from build123d import *

# Parameters (mm, degrees)
F0_W     = 12
F0_H     = 12
F1_DEPTH = 75
F2_R     = 3.6
F3_DEPTH = 80
F4_R     = 0.6


with BuildPart() as f1:
    # F0 (on Top) → F1 (new body)
    with BuildSketch(Plane.XY):
        Rectangle(F0_W, F0_H)
    extrude(amount=F1_DEPTH)

    # F2 (on face) → F3 (cut)
    with BuildSketch(Plane.XY.offset(75)):
        Circle(F2_R)
    extrude(amount=-F3_DEPTH, mode=Mode.SUBTRACT)

    # F4
    f4_edges = [f1.edges().sort_by_distance(p)[0] for p in [
        (-6, -6, 37.5),
        (6, -6, 37.5),
        (0, -6, 0),
        (0, -6, 75),
        (6, 6, 37.5),
        (6, 0, 0),
        (6, 0, 75),
        (-6, 6, 37.5),
        (0, 6, 0),
        (0, 6, 75),
        (-6, 0, 0),
        (-6, 0, 75),
    ]]
    fillet(f4_edges, radius=F4_R)


solid = f1.part
Read the model definition and answer for the solid it produces. Units are mm, in the model's axes. Coordinates: 2 decimals unless noted, no trailing zeros. Order: outer loops, then holes, each group sorted by start corner. A loop starts at its lowest first (then second) coordinate and runs counter-clockwise, first axis right, second up. Notation, with made-up numbers: (75.25, 7.5) - (119.25, 7.5) arc R36 ccw to (119.25, 42.5) - close; hole circle Ø3 at (34, 62.5). An arc over 180 degrees is marked (long way). Use one line per item in the form item = value.
(1) Section C-C, the plane z = 60.5 is taken. Give the vertices of the cut face in (x, y).
Computed values:
outline = (-6, -5.4) arc R0.6 ccw to (-5.4, -6) - (5.4, -6) arc R0.6 ccw to (6, -5.4) - (6, 5.4) arc R0.6 ccw to (5.4, 6) - (-5.4, 6) arc R0.6 ccw to (-6, 5.4) - close; hole circle Ø7.2 at (0, 0)
(2) Straight lines are drawn through the part: L1, parallel to Y at x = -0.25, z = 55; L2, parallel to Y at x = 2.25, z = 55; L3, parallel to X at y = 2.5, z = 47.5. For each, find the intervals that lie inside material, in ascending order.
Computed values:
L1 = -6 to -3.59, 3.59 to 6
L2 = -6 to -2.81, 2.81 to 6
L3 = -6 to -2.59, 2.59 to 6
(3) Section A-A, the plane x = 0 is taken. Give the vertices of the cut face in (y, z), then the cut area to 3 significant figures.
Computed values:
outline = (-6, 0.6) arc R0.6 ccw to (-5.4, 0) - (-3.6, 0) - (-3.6, 75) - (-5.4, 75) arc R0.6 ccw to (-6, 74.4) - close; (3.6, 0) - (5.4, 0) arc R0.6 ccw to (6, 0.6) - (6, 74.4) arc R0.6 ccw to (5.4, 75) - (3.6, 75) - close
area = 360 mm²
(4) For a pull along Y with two mould halves and no side action, classify faces 1 (the face through (0, 4, 0)), 2 (the face through (3.434, 1.081, 38.025)), 3 (the face through (0, -6, 37)) as pulls with the +Y half, pulls with the -Y half, needs draft (parallel to the pull), parting line crosses it, or undercut.
Computed values:
face_1 = needs draft
face_2 = undercut
face_3 = pulls with the -Y half
(5) Given pin 1 Ø2 at (x, y) = (-1, 4.5) entering from -Z; pin 2 Ø4.5 at (x, y) = (0, 0) entering from +Z, each flat-ended and moving along its own axis, determine where each tip first touches the part or whether it passes through.
Computed values:
pin_1 = 0
pin_2 = through
